Could you check a few things on this model? Use its own coordinates, in mm. Give positions to 0.01 mm unless a question says otherwise; leave off trailing zeros. Order: outer loops, then holes, each group sorted by start corner. A loop starts at its lowest first (then second) coordinate and runs counter-clockwise, first axis right, second up. Notation, with made-up numbers: (-37, 5.25) -> (7, 5.25) arc R24 cw to (7, 39.25) -> close; hole circle Ø7 at (56.5, -26). An arc over 180 degrees is marked (long way). Answer as CSV lines item,"result". Start each with the question number.
(1) I want a section at A-A (x = -24). Give the number of separate pieces and of enclosed holes in the cut face, plus the area to 3 significant figures.
(2) Will these pins go through, and if not, where does the flat tip stop? pin 1 Ø3 at (y, z) = (27, -1) entering from +X; pin 2 Ø3 at (y, z) = (-12.5, -1.5) entering from -X.
(3) I need wall thicknesses on L1, parallel to X at y = -21, z = -0.8; L2, parallel to Y at x = -24.5, z = -4.8; L3, parallel to X at y = 26, z = -3.8. Which ranges of each line are inside material? Lowest first, please.
(4) We'd pull the mould along Y, two halves only. Please class faces 1 (the face through (35.3, -27.01, -2.46)), 2 (the face through (-13.694, -32.131, -2.465)), 3 (the face through (44.116, 5.437, -2.465)): released by +Y, released by -Y, zero draft, split by the parting line, or undercut.
(5) I want a section at C-C (x = -10). Please give me the cut outline in (y, z).
(6) I want a section at D-D (y = 16). Please give me the cut outline in (x, z), plus the area to 3 significant figures.
```python
from build123d import *

# Parameters (mm, degrees)
F1_DEPTH = 5


with BuildPart() as f1:
    # F0 (on Top) → F1 (new body)
    with BuildSketch(Plane.XY):
        with BuildLine():
            add(Edge.make_bspline(
                [(17.960512809, -17.960512809), (15.6802243454, -20.2331445456), (29.0574428343, -33.6372935287)],
                knots=[6.282890907, 6.282890907, 6.282890907, 7.8477722056, 7.8477722056, 7.8477722056], degree=2, weights=[1, 0.7091949639, 1]))
            Line((17.960512809, -17.960512809), (4.4910260861, -4.4910260861))
            ThreePointArc((4.4910260861, -4.4910260861), (0, -6.35127), (-4.4910260861, -4.4910260861))
            Line((-4.4910260861, -4.4910260861), (-17.9660364379, -17.9660364379))
            add(Edge.make_bspline(
                [(-29.1037800474, -33.5972095114), (-15.9810329654, -20.44676612), (-17.9660364379, -17.9660364379)],
                knots=[1.576997225, 1.576997225, 1.576997225, 3.1227237577, 3.1227237577, 3.1227237577], degree=2, weights=[1, 0.7159145089, 1]))
            ThreePointArc((-29.1037800474, -33.5972095114), (-27.3554893491, -35.0354064122), (-25.5362426788, -36.3827268061))
            ThreePointArc((-25.5362426788, -36.3827268061), (-13.5131315962, -32.2048272696), (-8.0710910961, -43.7110968579))
            ThreePointArc((-8.0710910961, -43.7110968579), (-5.6632765753, -44.0877511156), (-3.2384377382, -44.3318736466))
            add(Edge.make_bspline(
                [(3.2384377382, -44.3318736466), (3.2184803968, -25.4), (0, -25.4), (-3.2184803968, -25.4), (-3.2384377382, -44.3318736466)],
                knots=[4.7185898786, 4.7185898786, 4.7185898786, 6.2831853072, 6.2831853072, 7.8477807358, 7.8477807358, 7.8477807358], degree=2, weights=[1, 0.7092957276, 1, 0.7092957276, 1]))
            ThreePointArc((3.2384377382, -44.3318736466), (5.6632776972, -44.0877509715), (8.0710933206, -43.7110964471))
            ThreePointArc((8.0710933206, -43.7110964471), (13.5131332351, -32.2048265819), (25.5362445304, -36.3827255066))
            ThreePointArc((25.5362445304, -36.3827255066), (27.3313377683, -35.0542504669), (29.0574428343, -33.6372935287))
        make_face()
        with BuildLine():
            add(Edge.make_bspline(
                [(44.3580588388, 2.8574667196), (25.4, 2.843741946), (25.4, 0), (25.4, -2.843741946), (44.3580588388, -2.8574667196)],
                knots=[4.7172153068, 4.7172153068, 4.7172153068, 6.2831853072, 6.2831853072, 7.8491553076, 7.8491553076, 7.8491553076], degree=2, weights=[1, 0.7088110847, 1, 0.7088110847, 1]))
            ThreePointArc((44.3580588388, 2.8574667196), (44.1116709386, 5.4738457236), (43.7110967552, 8.0710916523))
            ThreePointArc((43.7110967552, 8.0710916523), (32.2048270977, 13.5131320059), (36.3827264812, 25.5362431418))
            ThreePointArc((36.3827264812, 25.5362431418), (34.8720687583, 27.5634054594), (33.2486042571, 29.5014036099))
            add(Edge.make_bspline(
                [(18.0297160686, 18.0297160686), (19.9566530018, 15.2356768134), (33.2486042571, 29.5014036099)],
                knots=[3.1036959155, 3.1036959155, 3.1036959155, 4.6978570798, 4.6978570798, 4.6978570798], degree=2, weights=[1, 0.6987979995, 1]))
            Line((18.0297160686, 18.0297160686), (4.4910260861, 4.4910260861))
            ThreePointArc((4.4910260861, 4.4910260861), (5.8678083585, 2.4305258035), (6.35127, 0))
            ThreePointArc((6.35127, 0), (5.8678083585, -2.4305258035), (4.4910260861, -4.4910260861))
            Line((4.4910260861, -4.4910260861), (17.960512809, -17.960512809))
            add(Edge.make_bspline(
                [(33.6372860032, -29.0574515459), (20.2394978879, -15.6891800806), (17.960512809, -17.960512809)],
                knots=[4.7185813484, 4.7185813484, 4.7185813484, 6.282890907, 6.282890907, 6.282890907], degree=2, weights=[1, 0.7093964769, 1]))
            ThreePointArc((33.6372860032, -29.0574515459), (35.3259920878, -26.9791916672), (36.8864875406, -24.803014674))
            ThreePointArc((36.8864875406, -24.803014674), (32.4688107335, -12.8659222194), (43.8638664264, -7.1947009755))
            ThreePointArc((43.8638664264, -7.1947009755), (44.1642380736, -5.0321541488), (44.3580588388, -2.8574667196))
        make_face()
        with BuildLine():
            Line((4.4910260861, 4.4910260861), (18.0297160686, 18.0297160686))
            add(Edge.make_bspline(
                [(28.6070931031, 34.0211217362), (16.2285166945, 20.6414371225), (18.0297160686, 18.0297160686)],
                knots=[1.576997225, 1.576997225, 1.576997225, 3.1036959155, 3.1036959155, 3.1036959155], degree=2, weights=[1, 0.7225245136, 1]))
            ThreePointArc((28.6070931031, 34.0211217362), (26.7637763288, 35.4894741666), (24.8452280049, 36.8580675753))
            ThreePointArc((24.8452280049, 36.8580675753), (12.9030857851, 32.4540598727), (7.2449139151, 43.8556008095))
            ThreePointArc((7.2449139151, 43.8556008095), (5.247082468, 44.1392186788), (3.2384377382, 44.3318736466))
            add(Edge.make_bspline(
                [(-3.2384377382, 44.3318736466), (-3.2184803968, 25.4), (0, 25.4), (3.2184803968, 25.4), (3.2384377382, 44.3318736466)],
                knots=[1.576997225, 1.576997225, 1.576997225, 3.1415926536, 3.1415926536, 4.7061880822, 4.7061880822, 4.7061880822], degree=2, weights=[1, 0.7092957276, 1, 0.7092957276, 1]))
            ThreePointArc((-3.2384377382, 44.3318736466), (-5.6023539167, 44.0955341343), (-7.950266755, 43.7332340277))
            ThreePointArc((-7.950266755, 43.7332340277), (-13.4240835005, 32.2420471926), (-25.4356032496, 36.4531560682))
            ThreePointArc((-25.4356032496, 36.4531560682), (-27.2828792759, 35.091979118), (-29.0574503266, 33.6372870565))
            add(Edge.make_bspline(
                [(-17.9605125358, 17.9605125358), (-15.6879254577, 20.2386077571), (-29.0574503266, 33.6372870565)],
                knots=[0.0002118916, 0.0002118916, 0.0002118916, 1.5646015681, 1.5646015681, 1.5646015681], degree=2, weights=[1, 0.7093682423, 1]))
            Line((-17.9605125358, 17.9605125358), (-4.4910260861, 4.4910260861))
            ThreePointArc((-4.4910260861, 4.4910260861), (0, 6.35127), (4.4910260861, 4.4910260861))
        make_face()
        with BuildLine():
            ThreePointArc((-4.4910260861, -4.4910260861), (-6.35127, 0), (-4.4910260861, 4.4910260861))
            Line((-4.4910260861, 4.4910260861), (-17.9605125358, 17.9605125358))
            add(Edge.make_bspline(
                [(-33.6372924729, 29.0574440565), (-20.2340350033, 15.6814796579), (-17.9605125358, 17.9605125358)],
                knots=[4.7185960181, 4.7185960181, 4.7185960181, 6.2833971988, 6.2833971988, 6.2833971988], degree=2, weights=[1, 0.7092232054, 1]))
            ThreePointArc((-33.6372924729, 29.0574440565), (-35.0919796241, 27.2828786249), (-36.4531522707, 25.4356086919))
            ThreePointArc((-36.4531522707, 25.4356086919), (-32.2420451884, 13.4240883142), (-43.7332328408, 7.9502732843))
            ThreePointArc((-43.7332328408, 7.9502732843), (-44.0955337161, 5.6023572084), (-44.3318736466, 3.2384377382))
            add(Edge.make_bspline(
                [(-44.3318736466, -3.2384377382), (-25.4, -3.2184803968), (-25.4, 0), (-25.4, 3.2184803968), (-44.3318736466, 3.2384377382)],
                knots=[1.576997225, 1.576997225, 1.576997225, 3.1415926536, 3.1415926536, 4.7061880822, 4.7061880822, 4.7061880822], degree=2, weights=[1, 0.7092957276, 1, 0.7092957276, 1]))
            ThreePointArc((-44.3318736466, -3.2384377382), (-44.1564712104, -5.0998578651), (-43.9029457794, -6.9522551658))
            ThreePointArc((-43.9029457794, -6.9522551658), (-32.5393959561, -12.686344462), (-37.0229545531, -24.598848269))
            ThreePointArc((-37.0229545531, -24.598848269), (-35.4189008641, -26.8571026281), (-33.6773037539, -29.011061888))
            add(Edge.make_bspline(
                [(-17.9660364379, -17.9660364379), (-20.0264213053, -15.3910999362), (-33.6773037539, -29.011061888)],
                knots=[3.1227237577, 3.1227237577, 3.1227237577, 4.7057194921, 4.7057194921, 4.7057194921], degree=2, weights=[1, 0.7027805116, 1]))
            Line((-17.9660364379, -17.9660364379), (-4.4910260861, -4.4910260861))
        make_face()
    extrude(amount=-F1_DEPTH)


solid = f1.part
```
Final values:
1,separate pieces,"3"
1,enclosed holes,"0"
1,area,"268 mm²"
2,pin 1,"x = 36.38"
2,pin 2,"x = -33.4"
3,L1,"-33.22 to -24.6, -18.74 to 18.67, 24.5 to 33"
3,L2,"-34.87 to -28.69, -20.92 to 21, 28.78 to 35.06"
3,L3,"-36.05 to -30.45, -22.16 to -0.81, 0.81 to 21.91, 29.84 to 36.05"
4,face 1,"released by -Y"
4,face 2,"undercut"
4,face 3,"released by +Y"
5,outline,"(-34.75, -5) -> (34.67, -5) -> (34.67, 0) -> (-34.75, 0) -> close"
6,outline,"(-31.57, -5) -> (31.54, -5) -> (31.54, 0) -> (-31.57, 0) -> close"
6,area,"316 mm²"
